Geometry: final body of the model. Coordinates: model frame, mm. Face numbers are marked on the shaded views. A direction names the side the tool comes from. Give positions to 0.01 mm unless a question says otherwise; leave off trailing zeros. Write each loop counter-clockwise with the first axis right and the second up, starting at its lowest first coordinate (ties: lowest second). Pieces come first, ordered by that corner, then holes.
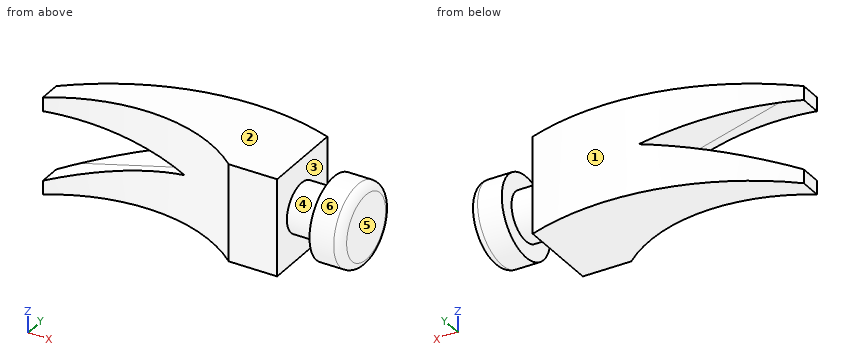
```python
from build123d import *

# Parameters (mm, degrees)
BOSS_EXTRUDE1_DEPTH = 60
CUT_EXTRUDE1_DEPTH  = 50
CUT_EXTRUDE2_DEPTH  = 50


with BuildPart() as part:
    # Sketch1 → Boss-Extrude1 (new body)
    with BuildSketch(Plane.XY):
        with BuildLine():
            Line((49.124764621, -30.033995939), (49.124764621, 21.387360298))
            ThreePointArc((49.124764621, 21.387360298), (-29.932176884, 27.124741995), (-100.875235379, -8.230597064))
            Line((-100.875235379, -8.230597064), (-100.875235379, -21.76381536))
            ThreePointArc((-100.875235379, -21.76381536), (-39.492781079, -5.839547279), (19.124764621, -30.033995939))
            Line((19.124764621, -30.033995939), (49.124764621, -30.033995939))
        make_face()
    extrude(amount=BOSS_EXTRUDE1_DEPTH)

    # Sketch3 → Revolve1 (revolve)
    with BuildSketch(Plane.XY.offset(30)):
        with BuildLine():
            Line((49.124764621, -5.033995939), (49.124764621, 9.966004061))
            Line((49.124764621, 9.966004061), (69.124764621, 9.966004061))
            Line((69.124764621, 9.966004061), (69.124764621, 19.966004061))
            Line((69.124764621, 19.966004061), (84.124764621, 19.966004061))
            ThreePointArc((84.124764621, 19.966004061), (87.660298526, 18.501537967), (89.124764621, 14.966004061))
            Line((89.124764621, 14.966004061), (89.124764621, -5.033995939))
            Line((89.124764621, -5.033995939), (49.124764621, -5.033995939))
        make_face()
    revolve(axis=Axis((49.124764621, -5.033995939, 30), (1, 0, 0)))

    # Sketch5 → Cut-Extrude1 (cut)
    with BuildSketch(Plane(origin=(0, 0, 0), x_dir=(1, 0, 0), z_dir=(0, 1, 0))):
        Polygon((-100.875235379, -8.547870984), (-100.875235379, -51.419743412), (-20.875235379, -30), align=None)
    extrude(amount=-CUT_EXTRUDE1_DEPTH, mode=Mode.SUBTRACT)

    # Sketch6 → Cut-Extrude2 (cut)
    with BuildSketch(Plane.XZ):
        Polygon((-90.829889616, 48.730134303), (-20.875235379, 30), (-90.829889616, 11.24154665), align=None)
    extrude(amount=-CUT_EXTRUDE2_DEPTH, mode=Mode.SUBTRACT)


solid = part.part
```
Item 1: Reachability of the marked faces 4, 5 and 6 from +Z, -Z, +X, -X, +Y, -Y: full face, straight path, thin tool, end or side. Return the list, or none.
Found:
face 4: none
face 5: +Z, -Z, +X, +Y, -Y
face 6: +X
Item 2: Section A-A, the plane x = -79.5. Return the cut outline in (y, z), plus the area to 3 significant figures.
Found:
outline: (-11.25, 0) - (7.71, 0) - (7.71, 14.28) - (-11.25, 14.28) - close; (-11.25, 45.7) - (7.71, 45.7) - (7.71, 60) - (-11.25, 60) - close
area: 542 mm2
Item 3: Section C-C, the plane x = 39.5. Return the cut outline in (y, z), plus the area to 3 significant figures.
Found:
outline: (-30.03, 0) - (24.43, 0) - (24.43, 60) - (-30.03, 60) - close
area: 3,270 mm2
Item 4: Pin query (flat end, axial travel): pin 1 Ø6 at (y, z) = (13.5, 9.5) entering from -X; pin 2 Ø8 at (y, z) = (-2, 50.5) entering from -X; pin 3 Ø2 at (y, z) = (5.5, 11.5) entering from -X; pin 4 Ø5 at (x, y) = (34, 0) entering from -Z. Return the tip coordinate at first contact, or that it passes through.
Found:
pin 1: stops at x = -74.77
pin 2: stops at x = -98.32
pin 3: stops at x = -84.49
pin 4: stops at z = 0
Item 5: Section B-B, the plane x = 72.5. Return the cut outline in (y, z), plus the area to 3 significant figures.
Found:
outline: circle Ø50 at (-5.03, 30)
area: 1,960 mm2
Item 6: Line query: L1, parallel to X at y = -19, z = 12.5; L2, parallel to X at y = -25, z = 15.5; L3, parallel to Z at x = -60.5, y = -0.5. Output: solid intervals per line, ascending.
Found:
L1: x = 3.63 to 49.12, 69.12 to 88.52
L2: x = 12.82 to 49.12, 69.12 to 85.9
L3: z = 0 to 19.37, 40.61 to 60
Item 7: Pull-direction query (X, two-part tool) for the marked faces 1, 2 and 3; classes: +X half, -X half, draft (parallel to the pull), parting line (faces both ways), or undercut.
Found:
face 1: parting line
face 2: draft
face 3: undercut
